The listing builds one solid part. Answer for the finished solid, in the listing's coordinates (mm). A direction names the side the tool comes from. Coordinates: 2 decimals unless noted, no trailing zeros. Order: outer loops, then holes, each group sorted by start corner. A loop starts at its lowest first (then second) coordinate and runs counter-clockwise, first axis right, second up.
```python
from build123d import *

# Parameters (mm, degrees)
SKETCH1_W           = 66
SKETCH1_H           = 17
SKETCH1_R           = 2
BOSS_EXTRUDE1_DEPTH = 1.2
SKETCH2_W           = 28
SKETCH2_H           = 2.54
BOSS_EXTRUDE2_DEPTH = 2
SKETCH3_R           = 0.5
BOSS_EXTRUDE3_DEPTH = 6


with BuildPart() as part:
    # Sketch1 → Boss-Extrude1 (new body)
    with BuildSketch(Plane(origin=(0, 0, 0), x_dir=(1, 0, 0), z_dir=(0, 1, 0))):
        Rectangle(SKETCH1_W, SKETCH1_H)
        with Locations((18.5, 4.5)):
            Circle(SKETCH1_R, mode=Mode.SUBTRACT)
        with Locations((-18.5, 4.5)):
            Circle(SKETCH1_R, mode=Mode.SUBTRACT)
    extrude(amount=BOSS_EXTRUDE1_DEPTH)

    # Sketch2 → Boss-Extrude2 (add)
    with BuildSketch(Plane(origin=(0, 1.2, 0), x_dir=(1, 0, 0), z_dir=(0, 1, 0))):
        with Locations((0, 6.5)):
            Rectangle(SKETCH2_W, SKETCH2_H)
    extrude(amount=BOSS_EXTRUDE2_DEPTH)

    # Sketch3 → Boss-Extrude3 (add)
    with BuildSketch(Plane(origin=(0, 3.2, 0), x_dir=(1, 0, 0), z_dir=(0, 1, 0))):
        with Locations((-12.73, 6.5)):
            Circle(SKETCH3_R)
        with Locations((-10.19, 6.5)):
            Circle(SKETCH3_R)
        with Locations((-7.65, 6.5)):
            Circle(SKETCH3_R)
        with Locations((-5.11, 6.5)):
            Circle(SKETCH3_R)
        with Locations((-2.57, 6.5)):
            Circle(SKETCH3_R)
        with Locations((-0.03, 6.5)):
            Circle(SKETCH3_R)
        with Locations((2.51, 6.5)):
            Circle(SKETCH3_R)
        with Locations((5.05, 6.5)):
            Circle(SKETCH3_R)
        with Locations((7.59, 6.5)):
            Circle(SKETCH3_R)
        with Locations((10.13, 6.5)):
            Circle(SKETCH3_R)
        with Locations((12.67, 6.5)):
            Circle(SKETCH3_R)
    extrude(amount=BOSS_EXTRUDE3_DEPTH)


solid = part.part
```
(1) Consider line 1 (X direction, y = 0.4, z = -4.5); line 2 (Z direction, x = 18.5, y = 0.55); line 3 (Y direction, x = -14.5, z = 5). Determine where each line is inside the solid, lowest interval first.
(2) For faces 5 (the face through (0, 2, -5.23)), 6 (the face through (14, 2, -6)), 7 (the face through (0, 2, -7.77)), 8 (the face through (-14, 2, -6)), determine the directions among +Z, -Z, +X, -X, +Y, -Y from which every point of the face is accessible in a straight line to the end or side of a thin tool.
(3) Each of these flat-tipped pins is pushed along its axis until it touches: pin 1 Ø2 at (y, z) = (2.5, -7) entering from -X; pin 2 Ø2 at (x, y) = (1, 2.5) entering from -Z; pin 3 Ø5 at (x, y) = (6.5, 4) entering from +Z. Where does it stop, or does it pass through?
(4) Find section C-C (z = 1.5). Write down the section's boundary in (x, y), and give its area (3 significant figures).
(5) Find section A-A (x = 18.5). Write down the section's boundary in (y, z), and give its area (3 significant figures).
(6) The mould has two halves that part along X. Classify faces 1 (the face through (-0.2, 3.2, -7.4)), 2 (the face through (0, 1, -8.5)), 3 (the face through (33, 1, 0)), 4 (the face through (-20.1, 0.6, -3.3)): released by +X, released by -X, zero draft, split by the parting line, or undercut.
(7) Find section B-B (y = 4.75). Give the number of separate pieces and of enclosed holes in the cut face, and give its area (3 significant figures).
Findings below:
1. line 1: x = -33 to -20.5, -16.5 to 16.5, 20.5 to 33
1. line 2: z = -8.5 to -6.5, -2.5 to 8.5
1. line 3: y = 0 to 1.2
2. face 5: +Z, +X, -X, +Y
2. face 6: +Z, -Z, +X, +Y
2. face 7: -Z, +X, -X, +Y
2. face 8: +Z, -Z, -X, +Y
3. pin 1: stops at x = -14
3. pin 2: stops at z = -7.77
3. pin 3: stops at z = -5.23
4. outline: (-33, 0) - (33, 0) - (33, 1.2) - (-33, 1.2) - close
4. area: 79.2 mm2
5. outline: (0, -8.5) - (1.2, -8.5) - (1.2, -6.5) - (0, -6.5) - close; (0, -2.5) - (1.2, -2.5) - (1.2, 8.5) - (0, 8.5) - close
5. area: 15.6 mm2
6. face 1: undercut
6. face 2: zero draft
6. face 3: released by +X
6. face 4: undercut
7. separate pieces: 11
7. enclosed holes: 0
7. area: 8.64 mm2
